Design review of the part built by this model. Coordinates are the model's own, in mm. Face numbers are marked on the shaded views. A direction names the side the tool comes from. Give positions to 0.01 mm unless a question says otherwise; leave off trailing zeros. Loops run counter-clockwise (first coordinate to the right, second up) from the corner with the lowest first, then second, coordinate; pieces in that order, holes last. Notation, with made-up numbers: (42.5, -20.75) -> (58.5, -20.75) arc R13 ccw to (58.5, 2.25) -> close; hole circle Ø6 at (-0.75, -1). An arc over 180 degrees is marked (long way). Use a Markdown table: item, result. Add a question column.
1. Draft analysis for pull direction Y (two halves, no side actions). For the marked faces 1, 2 and 3, state which applies: pulls with the +Y half, pulls with the -Y half, needs draft (parallel to the pull), parting line crosses it, or undercut.
2. Add section A-A (x = 0). State the section outline as (y, z) points, and give its area (3 significant figures).
3. For pin 1 Ø1.5 at (y, z) = (-157.5, 25) entering from -X; pin 2 Ø1 at (y, z) = (-21, 30.5) entering from -X; pin 3 Ø10 at (y, z) = (-141, 18) entering from +X; pin 4 Ø10 at (x, y) = (134, 36.5) entering from +Z, all flat-tipped, find the tip position at first contact; note any pin that passes through.
4. Add section C-C (z = 23). Count the separate pieces of the cut face and the enclosed holes in it, and give its area (3 significant figures).
5. Add section B-B (y = 0). State the section outline as (x, z) points.
6. To check wall thickness, follow line 1 (Y direction, x = 0, z = 15); line 2 (Y direction, x = 48.5, z = 27.5); line 3 (X direction, y = 24.5, z = 3). State the ranges of each line that lie inside material, in increasing order.
7. For the marked faces 4 and 5, list the 3-axis set-ups (+Z, -Z, +X, -X, +Y, -Y) from which the entire face can be reached by the end or side of a thin tool; tool diameter is ignored.
```python
from build123d import *

# Parameters (mm, degrees)
ESBO_O2_R             = 200
EXTRUS_O2_DEPTH       = 34
EXTRUS_O3_DEPTH       = 35
PADR_OCIRCULAR1_COUNT = 3
CASCA1_T              = -3
FILETE1_R             = 10
FILETE2_R             = 10
FILETE3_R             = 10
FILETE4_R             = 10
FILETE5_R             = 10
FILETE6_R             = 10
FILETE7_R             = 10
FILETE8_R             = 10
FILETE9_R             = 10
FILETE10_R            = 10
FILETE11_R            = 10
FILETE12_R            = 10
FILETE13_R            = 10
FILETE14_R            = 10
FILETE15_R            = 10
FILETE16_R            = 10
FILETE17_R            = 10
FILETE18_R            = 10
FILETE19_R            = 5


with BuildPart() as part:
    # Esboço2 → Extrusão2 (new body)
    with BuildSketch(Plane.XY):
        Circle(ESBO_O2_R)
    extrude(amount=EXTRUS_O2_DEPTH)

    # Esboço4 → Extrusão3 (cut, through all)
    with BuildSketch(Plane.XY.offset(34)):
        with BuildLine():
            Line((-103.980767452, -142), (103.980767452, -142))
            ThreePointArc((103.980767452, -142), (121.948545192, -126.903712812), (137.748134317, -109.551136426))
            Line((137.748134317, -109.551136426), (0, -30.022213998))
            Line((0, -30.022213998), (-137.748134317, -109.551136426))
            ThreePointArc((-137.748134317, -109.551136426), (-121.948545192, -126.903712812), (-103.980767452, -142))
        make_face()
    extrus_o3 = extrude(amount=-EXTRUS_O3_DEPTH, mode=Mode.SUBTRACT)

    # PadrãoCircular1: Extrusão3 ×3 about axis
    padr_ocircular1_axis = Axis((0, 0, 0), (0, 0, 1))
    for i in range(1, PADR_OCIRCULAR1_COUNT):
        add(extrus_o3.rotate(padr_ocircular1_axis, i * 360 / PADR_OCIRCULAR1_COUNT), mode=Mode.SUBTRACT)

    # Casca1
    casca1_openings = [part.faces().sort_by_distance(p)[0] for p in [
        (92.730670551, 53.538077605, 0),
    ]]
    offset(amount=CASCA1_T, openings=casca1_openings, kind=Kind.INTERSECTION)

    # Filete1
    filete1_edges = [part.edges().sort_by_distance(p)[0] for p in [
        (-137.748134317, -109.551136426, 17),
    ]]
    fillet(filete1_edges, radius=FILETE1_R)

    # Filete2
    filete2_edges = [part.edges().sort_by_distance(p)[0] for p in [
        (137.748134317, -109.551136426, 17),
    ]]
    fillet(filete2_edges, radius=FILETE2_R)

    # Filete3
    filete3_edges = [part.edges().sort_by_distance(p)[0] for p in [
        (-26, 174.068951855, 17),
    ]]
    fillet(filete3_edges, radius=FILETE3_R)

    # Filete4
    filete4_edges = [part.edges().sort_by_distance(p)[0] for p in [
        (-163.748134317, -64.517815429, 17),
    ]]
    fillet(filete4_edges, radius=FILETE4_R)

    # Filete5
    filete5_edges = [part.edges().sort_by_distance(p)[0] for p in [
        (26, 174.068951855, 17),
    ]]
    fillet(filete5_edges, radius=FILETE5_R)

    # Filete6
    filete6_edges = [part.edges().sort_by_distance(p)[0] for p in [
        (163.748134317, -64.517815429, 17),
    ]]
    fillet(filete6_edges, radius=FILETE6_R)

    # Filete7
    filete7_edges = [part.edges().sort_by_distance(p)[0] for p in [
        (0, -30.022213998, 17),
    ]]
    fillet(filete7_edges, radius=FILETE7_R)

    # Filete8
    filete8_edges = [part.edges().sort_by_distance(p)[0] for p in [
        (-26, 15.011106999, 17),
    ]]
    fillet(filete8_edges, radius=FILETE8_R)

    # Filete9
    filete9_edges = [part.edges().sort_by_distance(p)[0] for p in [
        (26, 15.011106999, 17),
    ]]
    fillet(filete9_edges, radius=FILETE9_R)

    # Filete10
    filete10_edges = [part.edges().sort_by_distance(p)[0] for p in [
        (-70.985223611, 161.049986119, 17),
    ]]
    fillet(filete10_edges, radius=FILETE10_R)

    # Filete11
    filete11_edges = [part.edges().sort_by_distance(p)[0] for p in [
        (-174.965991064, -19.049986119, 17),
    ]]
    fillet(filete11_edges, radius=FILETE11_R)

    # Filete12
    filete12_edges = [part.edges().sort_by_distance(p)[0] for p in [
        (-103.980767452, -142, 17),
    ]]
    fillet(filete12_edges, radius=FILETE12_R)

    # Filete13
    filete13_edges = [part.edges().sort_by_distance(p)[0] for p in [
        (103.980767452, -142, 17),
    ]]
    fillet(filete13_edges, radius=FILETE13_R)

    # Filete14
    filete14_edges = [part.edges().sort_by_distance(p)[0] for p in [
        (174.965991064, -19.049986119, 17),
    ]]
    fillet(filete14_edges, radius=FILETE14_R)

    # Filete15
    filete15_edges = [part.edges().sort_by_distance(p)[0] for p in [
        (70.985223611, 161.049986119, 17),
    ]]
    fillet(filete15_edges, radius=FILETE15_R)

    # Filete16
    filete16_edges = [part.edges().sort_by_distance(p)[0] for p in [
        (-142.233535704, -108.676682509, 15.5),
        (0, -26.558112383, 15.5),
        (-104.957134107, -145, 15.5),
        (-165.233535704, -68.839513935, 15.5),
        (-178.052250602, -18.395544445, 15.5),
        (-73.095116495, 163.395544445, 15.5),
        (165.233535704, -68.839513935, 15.5),
        (23, 13.279056191, 15.5),
        (23, 177.516196444, 15.5),
    ]]
    fillet(filete16_edges, radius=FILETE16_R)

    # Filete17
    filete17_edges = [part.edges().sort_by_distance(p)[0] for p in [
        (142.233535704, -108.676682509, 15.5),
        (104.957134107, -145, 15.5),
        (-23, 177.516196444, 15.5),
        (-23, 13.279056191, 15.5),
    ]]
    fillet(filete17_edges, radius=FILETE17_R)

    # Filete18
    filete18_edges = [part.edges().sort_by_distance(p)[0] for p in [
        (73.095116495, 163.395544445, 15.5),
        (178.052250602, -18.395544445, 15.5),
    ]]
    fillet(filete18_edges, radius=FILETE18_R)

    # Filete19
    filete19_edges = [part.edges().sort_by_distance(p)[0] for p in [
        (-200, 0, 34),
    ]]
    fillet(filete19_edges, radius=FILETE19_R)


solid = part.part
```
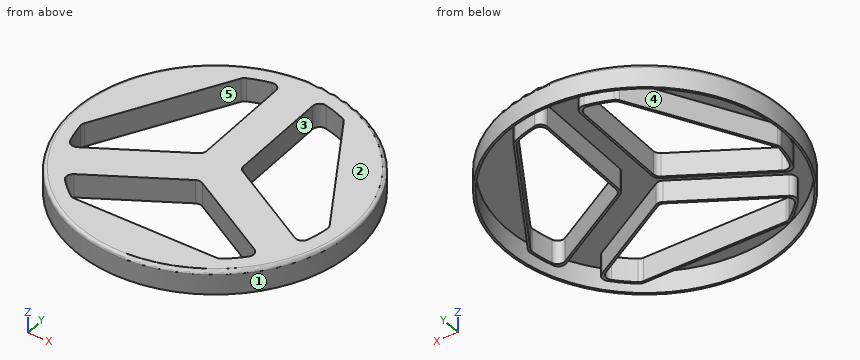
Taken from the geometry:
| question | item | result |
|---|---|---|
| 1 | face 1 | parting line crosses it |
| 1 | face 2 | needs draft |
| 1 | face 3 | undercut |
| 2 | outline | (-200, 0) -> (-197, 0) -> (-197, 31) -> (-145, 31) -> (-145, 0) -> (-142, 0) -> (-142, 34) -> (-195, 34) arc R5 ccw to (-200, 29) -> close; (-31.57, 0) -> (-28.11, 0) -> (-28.11, 31) -> (197, 31) -> (197, 0) -> (200, 0) -> (200, 29) arc R5 ccw to (195, 34) -> (-31.57, 34) -> close |
| 2 | area | 1,240 mm^2 |
| 3 | pin 1 | stops at x = -124.22 |
| 3 | pin 2 | stops at x = -198.81 |
| 3 | pin 3 | stops at x = 146.64 |
| 3 | pin 4 | passes through |
| 4 | separate pieces | 4 |
| 4 | enclosed holes | 4 |
| 4 | area | 9,430 mm^2 |
| 5 | outline | (-200, 0) -> (-197, 0) -> (-197, 31) -> (-167.43, 31) -> (-167.43, 0) -> (-163.97, 0) -> (-163.97, 34) -> (-195, 34) arc R5 ccw to (-200, 29) -> close; (-52, 0) -> (-46, 0) -> (-46, 31) -> (46, 31) -> (46, 0) -> (52, 0) -> (52, 34) -> (-52, 34) -> close; (163.97, 0) -> (167.43, 0) -> (167.43, 31) -> (197, 31) -> (197, 0) -> (200, 0) -> (200, 29) arc R5 ccw to (195, 34) -> (163.97, 34) -> close |
| 6 | line 1 | y = -200 to -197, -145 to -142, -31.57 to -28.11, 197 to 200 |
| 6 | line 2 | y = -194.03 to -190.94, -145 to -142, -58.02 to -54.56, -1.44 to 2.02, 169.19 to 172.3, 190.94 to 194.03 |
| 6 | line 3 | x = -198.49 to -195.47, -153.29 to -149.82, -26 to -23, 23 to 26, 149.82 to 153.29, 195.47 to 198.49 |
| 7 | face 4 | -Z |
| 7 | face 5 | +Z, -Z |
